Part model, mm, in its own coordinate system. Face numbers are marked on the shaded views. A direction names the side the tool comes from. Round coordinates to 2 decimals unless told otherwise and drop trailing zeros. Write each loop counter-clockwise with the first axis right and the second up, starting at its lowest first coordinate (ties: lowest second). Pieces come first, ordered by that corner, then holes.
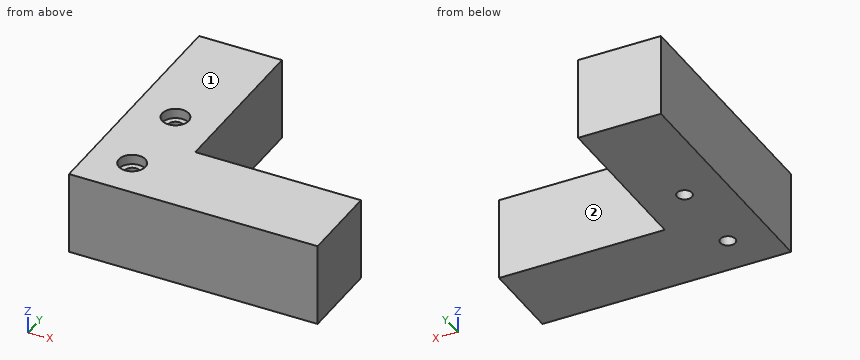
```python
from build123d import *

# Parameters (mm, degrees)
BOSS_EXTRUDE1_DEPTH = 25
SKETCH2_R           = 2.25
CUT_EXTRUDE1_DEPTH  = 25
SKETCH3_R           = 4
CUT_EXTRUDE2_DEPTH  = 3


with BuildPart() as part:
    # Sketch1 → Boss-Extrude1 (new body)
    with BuildSketch(Plane.XY):
        Polygon((-25, -25), (50, -25), (50, 0), (0, 0), (0, 50), (-25, 50), align=None)
    extrude(amount=BOSS_EXTRUDE1_DEPTH)

    # Sketch2 → Cut-Extrude1 (cut)
    with BuildSketch(Plane.XY.offset(25)):
        with Locations((-12.5, -12.5)):
            Circle(SKETCH2_R)
        with Locations((-12.5, 12.5)):
            Circle(SKETCH2_R)
    extrude(amount=-CUT_EXTRUDE1_DEPTH, mode=Mode.SUBTRACT)

    # Sketch3 → Cut-Extrude2 (cut)
    with BuildSketch(Plane.XY.offset(25)):
        with Locations((-12.5, 12.5)):
            Circle(SKETCH3_R)
        with Locations((-12.5, -12.5)):
            Circle(SKETCH3_R)
    extrude(amount=-CUT_EXTRUDE2_DEPTH, mode=Mode.SUBTRACT)


solid = part.part
```
Q1. Cut at B-B on x = -12.5. Write the cut outline in (y, z), plus the area to 3 significant figures.
Values follow:
outline: (-25, 0) - (-14.75, 0) - (-14.75, 22) - (-16.5, 22) - (-16.5, 25) - (-25, 25) - close; (-10.25, 0) - (10.25, 0) - (10.25, 22) - (8.5, 22) - (8.5, 25) - (-8.5, 25) - (-8.5, 22) - (-10.25, 22) - close; (14.75, 0) - (50, 0) - (50, 25) - (16.5, 25) - (16.5, 22) - (14.75, 22) - close
area: 1,630 mm2
Q2. Which spindle directions (+Z, -Z, +X, -X, +Y, -Y) get a long thin tool onto all of the face, cutting with end or side? Do the marked faces 1 and 2. Say none if no direction does.
Values follow:
face 1: +Z, +X, -X, +Y, -Y
face 2: +Z, -Z, +X, +Y
Q3. Cut at C-C on z = 3.25. Write the cut outline in (x, y), plus the area to 3 significant figures.
Values follow:
outline: (-25, -25) - (50, -25) - (50, 0) - (0, 0) - (0, 50) - (-25, 50) - close; hole circle Ø4.5 at (-12.5, -12.5); hole circle Ø4.5 at (-12.5, 12.5)
area: 3,090 mm2
Q4. Drop flat-ended pins along their axis: pin 1 (12.5 mm diameter, centred on x = 33, z = 17.5, fed in from +Y); pin 2 (12.5 mm diameter, centred on y = 33, z = 8.5, fed in from +X); pin 3 (2.5 mm diameter, centred on x = -11, y = -13.5, fed in from +Z). Give the stop position or say it passes through.
Values follow:
pin 1: stops at y = 0
pin 2: stops at x = 0
pin 3: stops at z = 22
Q5. Cut at D-D on y = 12.5. Write the cut outline in (x, z), plus the area to 3 significant figures.
Values follow:
outline: (-25, 0) - (-14.75, 0) - (-14.75, 22) - (-16.5, 22) - (-16.5, 25) - (-25, 25) - close; (-10.25, 0) - (0, 0) - (0, 25) - (-8.5, 25) - (-8.5, 22) - (-10.25, 22) - close
area: 502 mm2
Q6. Wall check: L1, parallel to Y at x = -12.5, z = 24.3; L2, parallel to Y at x = -12.5, z = 8.5; L3, parallel to X at y = 5.5, z = 3. Give the ranges that are in metal, low to high.
Values follow:
L1: y = -25 to -16.5, -8.5 to 8.5, 16.5 to 50
L2: y = -25 to -14.75, -10.25 to 10.25, 14.75 to 50
L3: x = -25 to 0
Q7. Cut at A-A on y = -12.5. Write the cut outline in (x, z), plus the area to 3 significant figures.
Values follow:
outline: (-25, 0) - (-14.75, 0) - (-14.75, 22) - (-16.5, 22) - (-16.5, 25) - (-25, 25) - close; (-10.25, 0) - (50, 0) - (50, 25) - (-8.5, 25) - (-8.5, 22) - (-10.25, 22) - close
area: 1,750 mm2
